Here's how the part is built. I have some questions about the finished solid (model axes, mm). Give positions to 0.01 mm unless a question says otherwise; leave off trailing zeros. Order: outer loops, then holes, each group sorted by start corner. A loop starts at its lowest first (then second) coordinate and runs counter-clockwise, first axis right, second up. Notation, with made-up numbers: (42, -23.75) -> (85, -23.75) arc R25 cw to (85, 5.25) -> close; hole circle Ø6 at (89, 16.5). An arc over 180 degrees is marked (long way). Write each question's results on one line, items separated by ' | '. Start each with the question number.
Q1. I'm going to push flat-ended pins straight in: pin 1 (2 mm diameter, centred on y = 0, z = 180, fed in from -X); pin 2 (12 mm diameter, centred on y = 0, z = 12.5, fed in from +X). Where does each tip first touch, or does it pass through?
Q2. Imagine slicing it at A-A, the plane z = -47.5. Please give me the cut outline in (x, y).
Q3. I need wall thicknesses on line 1 along Z through (x, y) = (-2.5, 0); line 2 along Y through (x, z) = (5, -47.5); line 3 along X through (y, z) = (-5, 187.5). Which ranges of each line are inside material? Lowest first, please. Write a range as [from, to].
```python
from build123d import *

# Parameters (mm, degrees)
SKETCH1_W               = 25
SKETCH1_H               = 25
BOSS_EXTRUDE1_DEPTH     = 200
SKETCH2_R               = 2.5
CUT_EXTRUDE1_DEPTH      = 202.943680268
SKETCH3_R               = 1.8
CUT_EXTRUDE2_DEPTH      = 202.943680268
SKETCH4_R               = 1.8
CUT_EXTRUDE3_DEPTH      = 202.943680268
CUT_EXTRUDE5_DEPTH      = 202.943680268
CUT_EXTRUDE5_DEPTH_BACK = 202.943680268
SKETCH6_R               = 2.5
CUT_EXTRUDE6_DEPTH      = 202.943680268
CUT_EXTRUDE6_DEPTH_BACK = 202.943680268
SKETCH7_R               = 5.3
CUT_EXTRUDE7_DEPTH      = 202.943680268
CUT_EXTRUDE7_DEPTH_BACK = 202.943680268
SKETCH8_W               = 75
SKETCH8_H               = 25


with BuildPart() as part:
    # Sketch1 → Boss-Extrude1 (new body)
    with BuildSketch(Plane.XY):
        Rectangle(SKETCH1_W, SKETCH1_H)
    boss_extrude1 = extrude(amount=BOSS_EXTRUDE1_DEPTH)

    # Sketch2 → Cut-Extrude1 (cut, through all)
    with BuildSketch(Plane(origin=(12.5, 0, 0), x_dir=(0, 0, -1), z_dir=(1, 0, 0))):
        with Locations(Location((-12.5, 0, 0), (0, 0, 90))):
            Circle(SKETCH2_R)
    cut_extrude1 = extrude(amount=-CUT_EXTRUDE1_DEPTH, mode=Mode.SUBTRACT)

    # Sketch3 → Cut-Extrude2 (cut, through all)
    with BuildSketch(Plane(origin=(0, 12.5, 0), x_dir=(1, 0, 0), z_dir=(0, 1, 0))):
        with Locations(Location((-5, -187.5, 0), (0, 0, 270))):
            Circle(SKETCH3_R)
        with Locations(Location((5, -187.5, 0), (0, 0, 270))):
            Circle(SKETCH3_R)
    cut_extrude2 = extrude(amount=-CUT_EXTRUDE2_DEPTH, mode=Mode.SUBTRACT)

    # Sketch4 → Cut-Extrude3 (cut, symmetric)
    with BuildSketch(Plane.ZY.offset(12.5)):
        with Locations(Location((180, 0, 0), (0, 0, 270))):
            Circle(SKETCH4_R)
    cut_extrude3 = extrude(amount=CUT_EXTRUDE3_DEPTH, both=True, mode=Mode.SUBTRACT)

    # Mirror2: Boss-Extrude1, Cut-Extrude1, Cut-Extrude2, Cut-Extrude3 across plane
    add(boss_extrude1.mirror(Plane(origin=(0, 0, 12.5), x_dir=(1, 0, 0), z_dir=(0, 0, -1))))
    add(cut_extrude1.mirror(Plane(origin=(0, 0, 12.5), x_dir=(1, 0, 0), z_dir=(0, 0, -1))), mode=Mode.SUBTRACT)
    add(cut_extrude2.mirror(Plane(origin=(0, 0, 12.5), x_dir=(1, 0, 0), z_dir=(0, 0, -1))), mode=Mode.SUBTRACT)
    add(cut_extrude3.mirror(Plane(origin=(0, 0, 12.5), x_dir=(1, 0, 0), z_dir=(0, 0, -1))), mode=Mode.SUBTRACT)

    # Sketch6 → Cut-Extrude5 (cut, two sides: drawn at the far end of the back side and taken through both)
    with BuildSketch(Plane(origin=(12.5, 0, 0), x_dir=(0, 0, -1), z_dir=(1, 0, 0)).offset(-CUT_EXTRUDE5_DEPTH_BACK)):
        with Locations(Location((7.5, 0, 0), (0, 0, 90))):
            Circle(SKETCH6_R)
        with Locations(Location((-12.5, 0, 0), (0, 0, 90))):
            Circle(SKETCH6_R)
        with Locations(Location((27.5, 0, 0), (0, 0, 90))):
            Circle(SKETCH6_R)
        with Locations(Location((47.5, 0, 0), (0, 0, 90))):
            Circle(SKETCH6_R)
    extrude(amount=CUT_EXTRUDE5_DEPTH + CUT_EXTRUDE5_DEPTH_BACK, mode=Mode.SUBTRACT)

    # Sketch7 → Cut-Extrude6 (cut, two sides: drawn at the far end of the back side and taken through both)
    with BuildSketch(Plane.ZY.offset(12.5).offset(-CUT_EXTRUDE6_DEPTH_BACK)):
        with Locations(Location((-47.5, 0, 0), (0, 0, 270))):
            Circle(SKETCH7_R)
        with Locations(Location((-27.5, 0, 0), (0, 0, 270))):
            Circle(SKETCH7_R)
        with Locations(Location((-7.5, 0, 0), (0, 0, 270))):
            Circle(SKETCH7_R)
        with Locations(Location((12.5, 0, 0), (0, 0, 270))):
            Circle(SKETCH7_R)
    extrude(amount=CUT_EXTRUDE6_DEPTH + CUT_EXTRUDE6_DEPTH_BACK, mode=Mode.SUBTRACT)

    # Sketch8 → Cut-Extrude7 (cut, two sides: drawn at the far end of the back side and taken through both)
    with BuildSketch(Plane.ZY.offset(12.5).offset(-CUT_EXTRUDE7_DEPTH_BACK)):
        with Locations((-137.5, 0)):
            Rectangle(SKETCH8_W, SKETCH8_H)
    extrude(amount=CUT_EXTRUDE7_DEPTH + CUT_EXTRUDE7_DEPTH_BACK, mode=Mode.SUBTRACT)


solid = part.part
```
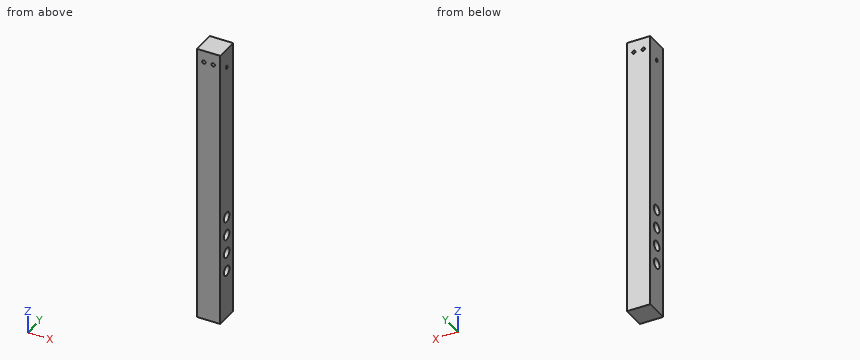
Geometry check:
1) pin 1: through | pin 2: x = 12.5
2) outline: (-12.5, -12.5) -> (12.5, -12.5) -> (12.5, -5.3) -> (-12.5, -5.3) -> close; (-12.5, 5.3) -> (12.5, 5.3) -> (12.5, 12.5) -> (-12.5, 12.5) -> close
3) line 1: [-100, -52.8], [-42.2, -32.8], [-22.2, -12.8], [-2.2, 7.2], [17.8, 178.2], [181.8, 200] | line 2: [-12.5, -5.3], [5.3, 12.5] | line 3: [-12.5, -6.8], [-3.2, 3.2], [6.8, 12.5]
